Design review of the part built by this model. Coordinates are the model's own, in mm. A direction names the side the tool comes from. Give positions to 0.01 mm unless a question says otherwise; leave off trailing zeros. Write each loop counter-clockwise with the first axis right and the second up, starting at its lowest first coordinate (ties: lowest second). Pieces come first, ordered by that corner, then holes.
```python
from build123d import *

# Parameters (mm, degrees)
F1_DEPTH  = 120
F2_R      = 2.65
F3_DEPTH  = 50
F4_DEPTH  = 11
F6_R      = 5
F6_R_2    = 2.65
F7_DEPTH  = 25
F10_DEPTH = 25
F11_W     = 11
F11_H     = 9
F12_DEPTH = 15.4995888315
F14_DEPTH = 100.001
F15_R     = 32.5
F16_DEPTH = 100
F17_R     = 27
F18_DEPTH = 3
F19_R     = 1
F20_DEPTH = 100.001
F21_R     = 67.5
F22_DEPTH = 50.001
F23_R     = 2


with BuildPart() as f1:
    # F0 (on Front) → F1 (new body)
    with BuildSketch(Plane.XZ):
        Polygon((-50, 0), (0, 0), (0, 50), (-33, 50), (-50, 10), align=None)
        Polygon((0, 50), (0, 0), (50, 0), (50, 10), (33, 50), align=None)
    extrude(amount=F1_DEPTH)

    # F2 (on Right) → F3 (cut, symmetric)
    with BuildSketch(Plane.YZ):
        with Locations((-35, 41.0004111685)):
            Circle(F2_R)
    extrude(amount=F3_DEPTH, both=True, mode=Mode.SUBTRACT)

    # F2 (on Right) → F4 (cut, symmetric)
    with BuildSketch(Plane.YZ):
        with BuildLine():
            Line((-22.5925706327, 34.5004111685), (0, 34.5004111685))
            Line((0, 34.5004111685), (0, 47.5004111685))
            Line((0, 47.5004111685), (-28.775050201, 47.5004111685))
            ThreePointArc((-28.775050201, 47.5004111685), (-26.7227858494, 44.5342088289), (-26, 41.0004111685))
            ThreePointArc((-26, 41.0004111685), (-26.7227858494, 37.4666135082), (-28.775050201, 34.5004111685))
            Line((-28.775050201, 34.5004111685), (-22.5925706327, 34.5004111685))
        make_face()
        with BuildLine():
            Line((-33.0777759178, 32.2080818652), (-22.5925706327, 34.5004111685))
            Line((-22.5925706327, 34.5004111685), (-28.775050201, 34.5004111685))
            ThreePointArc((-28.775050201, 34.5004111685), (-30.7682386679, 33.0573515547), (-33.0777759178, 32.2080818652))
        make_face()
        with BuildLine():
            Line((-28.775050201, 47.5004111685), (0, 47.5004111685))
            Line((0, 47.5004111685), (0, 56.6271956305))
            Line((0, 56.6271956305), (-27.1273270008, 51.5032727532))
            Line((-27.1273270008, 51.5032727532), (-35.0860282779, 50))
            ThreePointArc((-35.0860282779, 50), (-31.6858522299, 49.3679929314), (-28.775050201, 47.5004111685))
        make_face()
        with BuildLine():
            ThreePointArc((-33.0777759178, 32.2080818652), (-30.7682386679, 33.0573515547), (-28.775050201, 34.5004111685))
            ThreePointArc((-28.775050201, 34.5004111685), (-26.7227858494, 37.4666135082), (-26, 41.0004111685))
            ThreePointArc((-26, 41.0004111685), (-26.7227858494, 44.5342088289), (-28.775050201, 47.5004111685))
            ThreePointArc((-28.775050201, 47.5004111685), (-31.6858522299, 49.3679929314), (-35.0860282779, 50))
            ThreePointArc((-35.0860282779, 50), (-41.394304282, 47.3338835771), (-44, 41.0004111685))
            ThreePointArc((-44, 41.0004111685), (-40.6435796823, 33.9897044731), (-33.0777759178, 32.2080818652))
        make_face()
        with Locations((-35, 41.0004111685)):
            Circle(F2_R, mode=Mode.SUBTRACT)
        with BuildLine():
            Line((-44, 53.045399487), (-44, 41.0004111685))
            ThreePointArc((-44, 41.0004111685), (-41.394304282, 47.3338835771), (-35.0860282779, 50))
            Line((-35.0860282779, 50), (-27.1273270008, 51.5032727532))
            Line((-27.1273270008, 51.5032727532), (-44, 53.045399487))
        make_face()
    extrude(amount=F4_DEPTH, both=True, mode=Mode.SUBTRACT)

    # F6 (on offset) → F7 (cut)
    with BuildSketch(Plane.YZ.offset(24)):
        with Locations((-35, 41.0004111685)):
            Circle(F6_R)
        with Locations((-35, 41.0004111685)):
            Circle(F6_R_2, mode=Mode.SUBTRACT)
    extrude(amount=F7_DEPTH, mode=Mode.SUBTRACT)

    # F9 (on offset) → F10 (cut)
    with BuildSketch(Plane.YZ.offset(-30)):
        Polygon((-39.7920072343, 41.0004111685), (-37.3960036171, 36.8504111685), (-32.6039963829, 36.8504111685), (-30.2079927657, 41.0004111685), (-32.6039963829, 45.1504111685), (-37.3960036171, 45.1504111685), align=None)
    extrude(amount=-F10_DEPTH, mode=Mode.SUBTRACT)

    # F11 (on face) → F12 (cut, through all)
    with BuildSketch(Plane.XY.offset(50)):
        Polygon((-20, 0), (-11, -9), (-11, 0), align=None)
        Polygon((11, 0), (11, -9), (20, 0), align=None)
        with Locations((-5.5, -4.5)):
            Rectangle(F11_W, F11_H)
        with Locations((5.5, -4.5)):
            Rectangle(F11_W, F11_H)
    extrude(amount=-F12_DEPTH, mode=Mode.SUBTRACT)

    # F13 (on face) → F14 (cut, through all)
    with BuildSketch(Plane.YZ.offset(50)):
        Polygon((-105.143306435, 20), (-33.7286775579, 79.9239887514), (-151.3096454964, 75.0189004333), (-120, 37.7055179301), (-111.8561034844, 28), align=None)
        Polygon((-120, 28), (-111.8561034844, 28), (-120, 37.7055179301), align=None)
    extrude(amount=-F14_DEPTH, mode=Mode.SUBTRACT)

    # F15 (on face) → F16 (cut)
    with BuildSketch(Plane(origin=(0, -51.8525474655, -43.5094534539), x_dir=(-1, 0, 0), z_dir=(0, 0.7660444431, 0.6427876097))):
        with Locations((0, 103.0848769822)):
            Circle(F15_R)
    extrude(amount=F16_DEPTH, mode=Mode.SUBTRACT)

    # F17 (on face) → F18 (cut)
    with BuildSketch(Plane(origin=(0, -51.8525474655, -43.5094534539), x_dir=(-1, 0, 0), z_dir=(0, 0.7660444431, 0.6427876097))):
        with Locations((0, 103.0848769822)):
            Circle(F17_R)
    extrude(amount=-F18_DEPTH, mode=Mode.SUBTRACT)

    # F19 (on face) → F20 (cut, through all)
    with BuildSketch(Plane.YZ.offset(50)):
        with Locations((-20, 0)):
            Circle(F19_R)
        with Locations((-40, 0)):
            Circle(F19_R)
        with Locations((-60, 0)):
            Circle(F19_R)
        with Locations((-80, 0)):
            Circle(F19_R)
        with Locations((-100, 0)):
            Circle(F19_R)
    extrude(amount=-F20_DEPTH, mode=Mode.SUBTRACT)

    # F21 (on Top) → F22 (cut, through all)
    with BuildSketch(Plane.XY):
        with Locations((105, -60)):
            Circle(F21_R)
        with Locations((-105, -60)):
            Circle(F21_R)
    extrude(amount=F22_DEPTH, mode=Mode.SUBTRACT)

    # F23
    f23_edges = [f1.edges().sort_by_distance(p)[0] for p in [
        (20, 0, 42.250206),
        (11, -9, 42.250206),
        (-11, -9, 42.250206),
        (-25.476479, -87.267003, 35),
        (25.476479, -87.267003, 35),
        (0, -50.222895, 50),
        (-33.766783, -111.856103, 28),
        (33.766783, -111.856103, 28),
        (-35.613239, -105.143306, 20),
        (35.613239, -105.143306, 20),
        (0, -97.223632, 10.561699),
    ]]
    fillet(f23_edges, radius=F23_R)


solid = f1.part
```
(1) Consider section C-C, the plane x = 29. Give the boundary of the cut face in (y, z).
Resolved:
outline: (-120, 0) - (-101, 0) arc R1 cw to (-99, 0) - (-81, 0) arc R1 cw to (-79, 0) - (-61, 0) arc R1 cw to (-59, 0) - (-41, 0) arc R1 cw to (-39, 0) - (-21, 0) arc R1 cw to (-19, 0) - (0, 0) - (0, 50) - (-69.39, 50) - (-103.61, 21.29) arc R2 cw to (-106.43, 21.53) - (-111.26, 27.29) arc R2 ccw to (-112.79, 28) - (-120, 28) - close; hole circle Ø10 at (-35, 41)
(2) Mouldability with a two-part tool opening along Z and no side actions: class faces 1 (the face through (-32, -35, 45.15)), 2 (the face through (-1, -120, 14)), 3 (the face through (35.813, -105.093, 20.827)) as pulls with the +Z half, pulls with the -Z half, needs draft (parallel to the pull), parting line crosses it, or undercut.
Resolved:
face 1: undercut
face 2: needs draft
face 3: pulls with the +Z half
(3) Tool access review of faces 4 (the face through (33.86, -90.543, 32.251)), 5 (the face through (0.4, -73, 30.89)), 6 (the face through (-32.61, -38.58, 43.1)), 7 (the face through (-16, -4, 42)): name each direction out of +Z, -Z, +X, -X, +Y, -Y from which nothing blocks a thin tool from reaching the whole face with its end or side.
Resolved:
face 4: +Z, +X, -X
face 5: +Z
face 6: -X
face 7: +Z, +Y
(4) Consider section A-A, the plane y = -35. Give the boundary of the cut face in (x, z), then the cut area to 3 significant figures.
Resolved:
outline: (-42.3, 0) - (42.3, 0) - (42.3, 28.12) - (38.95, 36) - (24, 36) - (24, 38.35) - (11, 38.35) - (11, 32) - (-11, 32) - (-11, 38.35) - (-30, 38.35) - (-30, 36.85) - (-38.59, 36.85) - (-42.3, 28.12) - close; (-35.06, 45.15) - (-30, 45.15) - (-30, 43.65) - (-11, 43.65) - (-11, 50) - (-33, 50) - close; (11, 43.65) - (24, 43.65) - (24, 46) - (34.7, 46) - (33, 50) - (11, 50) - close
area: 3,280 mm2
(5) Clearance check with flat-ended pins moving along their axes: P1, Ø13, axis at y = -35, z = 41, coming from the -X side; P2, Ø12, axis at y = -46.5, z = 31, coming from the -X side; P3, Ø2, axis at x = 15.5, y = -65.5, coming from the +Z side; P4, Ø3, axis at y = -35, z = 41, coming from the -X side. State where each tip first meets the part, or that it passes through.
Resolved:
P1: stops at x = -39.59
P2: stops at x = -40.38
P3: stops at z = 43.43
P4: passes through
(6) To check wall thickness, follow L1, parallel to Z at x = 32.25, y = -35; L2, parallel to Z at x = 16, y = -35; L3, parallel to Z at x = 35.25, y = -35. State the ranges of each line that lie inside material, in increasing order.
Resolved:
L1: z = 0 to 36, 46 to 50
L2: z = 0 to 38.35, 43.65 to 50
L3: z = 0 to 36
(7) Consider section B-B, the plane z = 8. Give the boundary of the cut face in (x, y), then the cut area to 3 significant figures.
Resolved:
outline: (-50, -120) - (50, -120) - (50, -99.13) arc R67.5 cw to (50, -20.87) - (50, 0) - (-50, 0) - (-50, -20.87) arc R67.5 cw to (-50, -99.13) - close
area: 10,700 mm2
